Geometry check sheet. Reference: the model listing, model coordinates, mm. A direction names the side the tool comes from. Coordinates: 2 decimals unless noted, no trailing zeros. Write each loop counter-clockwise with the first axis right and the second up, starting at its lowest first coordinate (ties: lowest second). Pieces come first, ordered by that corner, then holes. Notation, with made-up numbers: (77.25, 38) -> (133.25, 38) arc R33 ccw to (133.25, 74) -> close; hole circle Ø8 at (-23.5, 35). An arc over 180 degrees is marked (long way). Answer in a Markdown table with one row per item. Add a question column.
Q1. Section check C-C, the plane z = 23.5. Record the boundary of the cut face in (x, y), and give its area (3 significant figures).
Q2. Section check D-D, the plane y = 6. Count the separate pieces of the cut face and the enclosed holes in it, and give its area (3 significant figures).
Q3. Gauge pin test, flat ends, axial feed: P1, Ø6.5, axis at x = 0, z = 0, coming from the +Y side; P2, Ø2, axis at y = 6, z = -12, coming from the +X side; P3, Ø7, axis at x = 9.5, z = 33, coming from the -Y side; P4, Ø1.5, axis at x = 57, z = -1, coming from the +Y side. Record the tip position at first contact, or that the pin passes through.
Q4. Tool access check on faces 5 (the face through (56, 10, 0)), 6 (the face through (4.6, 2.5, -20)), 7 (the face through (51, 6, 0)), 8 (the face through (-57, 10, 0)), 9 (the face through (-54.73, 4.78, -12.27)). Record the directions out of +Z, -Z, +X, -X, +Y, -Y that give a thin tool (end or side, any length) a straight path to the whole face; none if there is none.
Q5. Release check for a two-part mould opening along X. For faces 1 (the face through (-58, 5, 0)), 2 (the face through (58, 5, 0)), 3 (the face through (-54.73, 4.78, 11.73)), 4 (the face through (-1, 3, 4)) record: pulls with the +X half, pulls with the -X half, needs draft (parallel to the pull), parting line crosses it, or undercut.
Q6. Section check A-A, the plane x = 0. Record the boundary of the cut face in (y, z).
Q7. Thickness scan on line 1 (Z direction, x = -52.5, y = 6); line 2 (Y direction, x = -55, z = 12); line 3 (Y direction, x = -52, z = -12). Record the ranges inside material, lowest first.
Q8. Section check B-B, the plane y = 11.75. Record the boundary of the cut face in (x, z).
```python
from build123d import *
from build123d.topology import SkipClean

# Parameters (mm, degrees)
SKETCH_1_W               = 116
SKETCH_1_H               = 40
EXTRUDE_1_DEPTH          = 3
SKETCH_2_R               = 2.5
CUT_EXTRUDE_1_DEPTH      = 3
SKETCH_3_W               = 3
SKETCH_3_H               = 40
EXTRUDE_2_DEPTH          = 7
CHAMFER_1_SIZE           = 7
CUT_EXTRUDE_2_DEPTH      = 119.135515405
CUT_EXTRUDE_2_DEPTH_BACK = 119.135515405
SKETCH_4_R               = 1.25
SKETCH_6_R               = 43
SKETCH_6_R_2             = 40
EXTRUDE_1_2_DEPTH        = 3
EXTRUDE_3_DEPTH          = 17


with BuildPart() as part:
    # Sketch 1 → Extrude 1 (new body)
    with BuildSketch(Plane(origin=(0, 0, 0), x_dir=(1, 0, 0), z_dir=(0, 1, 0))):
        Rectangle(SKETCH_1_W, SKETCH_1_H)
    extrude(amount=EXTRUDE_1_DEPTH)

    # Sketch 2 → Cut-Extrude 1 (cut)
    with BuildSketch(Plane(origin=(0, 3, 0), x_dir=(1, 0, 0), z_dir=(0, 1, 0))):
        with Locations(Location((0, 0, 0), (0, 0, 270))):
            Circle(SKETCH_2_R)
    extrude(amount=-CUT_EXTRUDE_1_DEPTH, mode=Mode.SUBTRACT)

    # Sketch 3 → Extrude 2 (add)
    with BuildSketch(Plane(origin=(0, 3, 0), x_dir=(1, 0, 0), z_dir=(0, 1, 0))):
        with Locations((-56.5, 0)):
            Rectangle(SKETCH_3_W, SKETCH_3_H)
        with Locations((56.5, 0)):
            Rectangle(SKETCH_3_W, SKETCH_3_H)
    extrude(amount=EXTRUDE_2_DEPTH)

    # Chamfer 1
    chamfer_1_edges = [part.edges().sort_by_distance(p)[0] for p in [
        (-55, 3, 0),
        (55, 3, 0),
    ]]
    chamfer(chamfer_1_edges, length=CHAMFER_1_SIZE - 0.0001)  # a hair under: the kernel refuses the full size

    # Sketch 4 → Cut-Extrude 2 (cut, two sides: drawn at the far end of the back side and taken through both)
    with BuildSketch(Plane.ZY.offset(58).offset(-CUT_EXTRUDE_2_DEPTH_BACK)):
        with Locations((-12, 6)):
            Circle(SKETCH_4_R)
        with Locations((12, 6)):
            Circle(SKETCH_4_R)
    extrude(amount=CUT_EXTRUDE_2_DEPTH + CUT_EXTRUDE_2_DEPTH_BACK, mode=Mode.SUBTRACT)



with BuildPart() as body_2:
    # Sketch 6 → Extrude 1 2 (new body)
    with BuildSketch(Plane(origin=(0, 23, 0), x_dir=(1, 0, 0), z_dir=(0, 1, 0))):
        Circle(SKETCH_6_R)
        Circle(SKETCH_6_R_2, mode=Mode.SUBTRACT)
    extrude(amount=-EXTRUDE_1_2_DEPTH)


with BuildPart() as part_1:
    with SkipClean():  # the faces are left unmerged after this step: merging them gives an invalid solid
        add(part.part)

        add(body_2.part)  # Extrude 3 merges body 2
        # Sketch 7 → Extrude 3 (add)
        with BuildSketch(Plane(origin=(0, 3, 0), x_dir=(1, 0, 0), z_dir=(0, 1, 0))):
            with BuildLine():
                Line((-34.641016151, 20), (-38.065732621, 20))
                ThreePointArc((-38.065732621, 20), (-43, 0), (-38.065732621, -20))
                Line((-38.065732621, -20), (-34.641016151, -20))
                ThreePointArc((-34.641016151, -20), (-40, 0), (-34.641016151, 20))
            make_face()
            with BuildLine():
                ThreePointArc((43, 0), (41.748212553, 10.299842166), (38.065732621, 20))
                Line((38.065732621, 20), (34.641016151, 20))
                ThreePointArc((34.641016151, 20), (38.637033052, 10.352761804), (40, 0))
                ThreePointArc((40, 0), (38.637033052, -10.352761804), (34.641016151, -20))
                Line((34.641016151, -20), (38.065732621, -20))
                ThreePointArc((38.065732621, -20), (41.748212553, -10.299842166), (43, 0))
            make_face()
        extrude(amount=EXTRUDE_3_DEPTH)


solid = part_1.part
```
Calculated:
| question | item | result |
|---|---|---|
| 1 | outline | (-36.01, 20) -> (-32.37, 20) -> (-32.37, 23) -> (-36.01, 23) -> close; (32.37, 20) -> (36.01, 20) -> (36.01, 23) -> (32.37, 23) -> close |
| 1 | area | 21.8 mm² |
| 2 | separate pieces | 8 |
| 2 | enclosed holes | 0 |
| 2 | area | 740 mm² |
| 3 | P1 | stops at y = 3 |
| 3 | P2 | stops at x = 41.57 |
| 3 | P3 | passes through |
| 3 | P4 | stops at y = 10 |
| 4 | face 5 | +Z, -Z, +X, +Y |
| 4 | face 6 | -Z, +X, -X, -Y |
| 4 | face 7 | +Z, -Z, +Y |
| 4 | face 8 | +Z, -Z, -X, +Y |
| 4 | face 9 | -X |
| 5 | face 1 | pulls with the -X half |
| 5 | face 2 | pulls with the +X half |
| 5 | face 3 | needs draft |
| 5 | face 4 | undercut |
| 6 | outline | (0, -20) -> (3, -20) -> (3, -2.5) -> (0, -2.5) -> close; (0, 2.5) -> (3, 2.5) -> (3, 20) -> (0, 20) -> close; (20, -43) -> (23, -43) -> (23, -40) -> (20, -40) -> close; (20, 40) -> (23, 40) -> (23, 43) -> (20, 43) -> close |
| 7 | line 1 | z = -20 to -13.25, -10.75 to 10.75, 13.25 to 20 |
| 7 | line 2 | y = 0 to 4.75, 7.25 to 10 |
| 7 | line 3 | y = 0 to 4.75 |
| 8 | outline | (-38.07, -20) -> (-34.64, -20) arc R40 cw to (-34.64, 20) -> (-38.07, 20) arc R43 ccw to start; (34.64, -20) -> (38.07, -20) arc R43 ccw to (38.07, 20) -> (34.64, 20) arc R40 cw to start |
